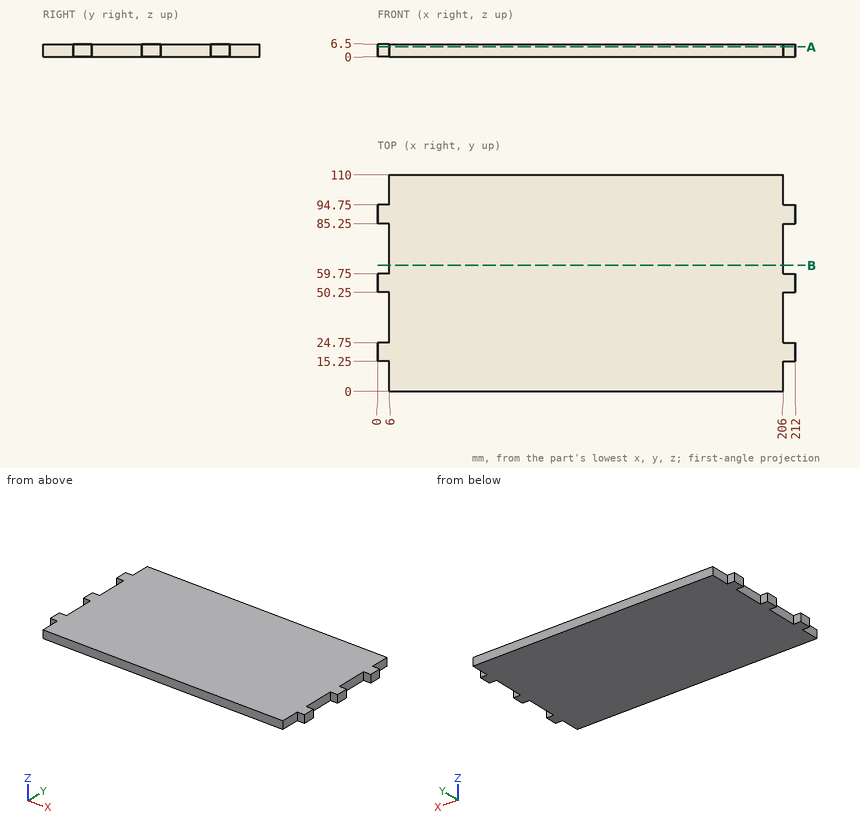
Input: dimensioned drawing with shaded views. Units: mm. Origin: part minimum x, y, z. Give positions to 0.01 mm unless a question says otherwise; leave off trailing zeros. Write each loop counter-clockwise with the first axis right and the second up, starting at its lowest first coordinate (ties: lowest second). Pieces come first, ordered by that corner, then holes. Notation, with made-up numbers: M 35,56.5 L 39,56.5 A11 ccw 39,67.5 Z; hole C 42.5,47 d10. An arc over 180 degrees is marked long. Return JSON: item names as keys, results as strings. Group by question number.
1) Pin query (flat end, axial travel): P1, Ø1, axis at y = 40, z = 2.5, coming from the +X side; P2, Ø1.8, axis at x = 2, z = 2.5, coming from the +Y side; P3, Ø1.8, axis at x = 209.5, z = 2.5, coming from the -Y side. Return the tip coordinate at first contact, or that it passes through.
2) Material intervals for line 1 along X through (y, z) = (62, 2.75), sorted ascending. Write a range as [from, to].
3) Cut plane A-A, the plane z = 5. Output: boundary loops of the cut face in (x, y).
4) Cut plane B-B, the plane y = 64. Output: boundary loops of the cut face in (x, z), plus the area to 3 significant figures.
Recorded:
{
 "1": {"P1": "stops at x = 206", "P2": "stops at y = 94.75", "P3": "stops at y = 15.25"},
 "2": {"line 1": "x = [6, 206]"},
 "3": {"outline": "M 0,15.25 L 6,15.25 L 6,0 L 206,0 L 206,15.25 L 212,15.25 L 212,24.75 L 206,24.75 L 206,50.25 L 212,50.25 L 212,59.75 L 206,59.75 L 206,85.25 L 212,85.25 L 212,94.75 L 206,94.75 L 206,110 L 6,110 L 6,94.75 L 0,94.75 L 0,85.25 L 6,85.25 L 6,59.75 L 0,59.75 L 0,50.25 L 6,50.25 L 6,24.75 L 0,24.75 Z"},
 "4": {"outline": "M 6,0 L 206,0 L 206,6.5 L 6,6.5 Z", "area": "1,300 mm²"}
}
